from build123d import *

# Parameters (mm, degrees)
ESQUISSE1_R             = 6
BOSS_EXTRU_1_DEPTH      = 190
BOSS_EXTRU_2_DEPTH      = 20
BOSS_EXTRU_3_START      = 20
BOSS_EXTRU_3_DEPTH      = 20
BOSS_EXTRU_5_DEPTH      = 8
BOSS_EXTRU_5_DEPTH_BACK = 8
ESQUISSE5_W             = 84
ESQUISSE5_H             = 12


with BuildPart() as part:
    # Esquisse1 → Boss.-Extru.1 (new body)
    with BuildSketch(Plane.XY):
        Circle(ESQUISSE1_R)
    extrude(amount=BOSS_EXTRU_1_DEPTH)

    # Esquisse2 → Boss.-Extru.2 (add)
    with BuildSketch(Plane.XY.offset(190)):
        with BuildLine():
            Line((-1, 1.5), (1, 1.5))
            ThreePointArc((1, 1.5), (2.5, 0), (1, -1.5))
            Line((1, -1.5), (-1, -1.5))
            ThreePointArc((-1, -1.5), (-2.5, 0), (-1, 1.5))
        make_face()
    extrude(amount=BOSS_EXTRU_2_DEPTH)

    # Esquisse3 → Boss.-Extru.3 (add)
    with BuildSketch(Plane(origin=(0, 0, 0), x_dir=(-1, 0, 0), z_dir=(0, 0, -1)).offset(BOSS_EXTRU_3_START)):
        with BuildLine():
            Line((-1, 1.5), (1, 1.5))
            ThreePointArc((1, 1.5), (2.5, 0), (1, -1.5))
            Line((1, -1.5), (-1, -1.5))
            ThreePointArc((-1, -1.5), (-2.5, 0), (-1, 1.5))
        make_face()
    extrude(amount=-BOSS_EXTRU_3_DEPTH)

    # Esquisse5 → Boss.-Extru.5 (add, two sides: drawn at the far end of the back side and taken through both)
    with BuildSketch(Plane(origin=(0, 0, 0), x_dir=(0, 0, -1), z_dir=(-1, 0, 0)).offset(-BOSS_EXTRU_5_DEPTH_BACK)):
        with Locations((-95, 0)):
            Rectangle(ESQUISSE5_W, ESQUISSE5_H)
    extrude(amount=BOSS_EXTRU_5_DEPTH + BOSS_EXTRU_5_DEPTH_BACK)


solid = part.part
Can you work these out from the model? Positions are in its coordinate system, mm. A direction names the side the tool comes from. Give positions to 0.01 mm unless a question says otherwise; leave off trailing zeros. Order: outer loops, then holes, each group sorted by start corner. A loop starts at its lowest first (then second) coordinate and runs counter-clockwise, first axis right, second up. Notation, with made-up numbers: M 55,4.5 L 87,4.5 A13 ccw 87,18.5 Z; hole C 49,80.5 d9. An arc over 180 degrees is marked long. One line per item, written item: value.
Item 1: For faces 1 (the face through (3, 0, 0)), 2 (the face through (-7, 0, 53)), 3 (the face through (-6, 0, 163)), 4 (the face through (-7, 0, 137)), which set-ups out of +Z, -Z, +X, -X, +Y, -Y let a thin tool reach every point of the face, with its end or its side?
Verdict:
face 1: -Z
face 2: -Z, -X
face 3: +Z
face 4: +Z, -X
Item 2: Please list where these lines run through material, in increasing order: line 1 (Z direction, x = -6.75, y = -1.75); line 2 (Y direction, x = 0.75, z = -10); line 3 (X direction, y = 0.25, z = 6).
Verdict:
line 1: 53 to 137
line 2: -1.5 to 1.5
line 3: -5.99 to 5.99
Item 3: For pin 1 (1 mm diameter, centred on x = 0, z = -5.5, fed in from -Y); pin 2 (2 mm diameter, centred on x = 0.5, z = -6.5, fed in from +Y); pin 3 (4 mm diameter, centred on x = -5.5, y = -1, fed in from -Z), each with a flat end and sliding along its axis, tell me the tip position at first contact or that it passes through.
Verdict:
pin 1: y = -1.5
pin 2: y = 1.5
pin 3: z = 0
Item 4: If we section it at A-A on z = 139: Write out the boundary of the cut face in (x, y).
Verdict:
outline: C 0,0 d12
Item 5: If we section it at B-B on y = 4: Write out the boundary of the cut face in (x, z), and give its area (3 significant figures).
Verdict:
outline: M -8,53 L -4.47,53 L -4.47,0 L 4.47,0 L 4.47,53 L 8,53 L 8,137 L 4.47,137 L 4.47,190 L -4.47,190 L -4.47,137 L -8,137 Z
area: 2,290 mm2
